```python
from build123d import *

# Parameters (mm, degrees)
F0_W      = 460
F0_H      = 450
F1_DEPTH  = 10
F2_R      = 2.5
F3_DEPTH  = 23
F4_W      = 40
F4_H      = 220
F5_DEPTH  = 160
F6_W      = 380
F6_H      = 25
F7_DEPTH  = 60
F8_W      = 58
F8_H      = 21
F9_DEPTH  = 382.2
F10_DEPTH = 401
F11_W     = 25
F11_H     = 387.5
F12_DEPTH = 60
F13_W     = 21
F13_H     = 58
F14_DEPTH = 386.4
F15_W     = 58
F15_H     = 25
F16_DEPTH = 3.3
F17_W     = 365
F17_H     = 25
F18_DEPTH = 60
F19_W     = 58
F19_H     = 21
F20_DEPTH = 366.6


with BuildPart() as f1:
    # F0 (on Front) → F1 (new body)
    with BuildSketch(Plane.XZ):
        Rectangle(F0_W, F0_H)
    extrude(amount=F1_DEPTH)

    # F2 (on face) → F3 (cut)
    with BuildSketch(Plane.XZ.offset(10)):
        with Locations((210, 205)):
            Circle(F2_R)
        with Locations((-210, 205)):
            Circle(F2_R)
        with Locations((-210, -205)):
            Circle(F2_R)
        with Locations((210, -205)):
            Circle(F2_R)
    extrude(amount=-F3_DEPTH, mode=Mode.SUBTRACT)

    # F4 (on face) → F5 (join)
    with BuildSketch(Plane.XZ.offset(10)):
        with Locations((-195, 60)):
            Rectangle(F4_W, F4_H)
    extrude(amount=F5_DEPTH)

    # F6 (on face) → F7 (join)
    with BuildSketch(Plane.XZ.offset(10)):
        with Locations((0, 202.5)):
            Rectangle(F6_W, F6_H)
        with Locations((0, -202.5)):
            Rectangle(F6_W, F6_H)
    extrude(amount=F7_DEPTH)

    # F8 (on face) → F9 (cut)
    with BuildSketch(Plane.YZ.offset(190)):
        with Locations((-41, 202.5)):
            Rectangle(F8_W, F8_H)
    extrude(amount=-F9_DEPTH, mode=Mode.SUBTRACT)

    # F8 (on face) → F10 (cut)
    with BuildSketch(Plane.YZ.offset(190)):
        with Locations((-41, -202.5)):
            Rectangle(F8_W, F8_H)
    extrude(amount=-F10_DEPTH, mode=Mode.SUBTRACT)

    # F11 (on face) → F12 (join)
    with BuildSketch(Plane.XZ.offset(10)):
        with Locations((210.504704, -3.75)):
            Rectangle(F11_W, F11_H)
    extrude(amount=F12_DEPTH)

    # F13 (on face) → F14 (cut)
    with BuildSketch(Plane(origin=(0, 0, -197.5), x_dir=(1, 0, 0), z_dir=(0, 0, -1))):
        with Locations((210.504704, 41)):
            Rectangle(F13_W, F13_H)
    extrude(amount=-F14_DEPTH, mode=Mode.SUBTRACT)

    # F15 (on face) → F16 (cut)
    with BuildSketch(Plane(origin=(198.004704, 0, 0), x_dir=(0, -1, 0), z_dir=(-1, 0, 0))):
        with Locations((41, -44.218161)):
            Rectangle(F15_W, F15_H)
    extrude(amount=-F16_DEPTH, mode=Mode.SUBTRACT)

    # F17 (on face) → F18 (join)
    with BuildSketch(Plane.XZ.offset(10)):
        with Locations((13.504704, -44.218161)):
            Rectangle(F17_W, F17_H)
    extrude(amount=F18_DEPTH)

    # F19 (on face) → F20 (cut)
    with BuildSketch(Plane.YZ.offset(196.004704)):
        with Locations((-41, -44.218161)):
            Rectangle(F19_W, F19_H)
    extrude(amount=-F20_DEPTH, mode=Mode.SUBTRACT)


solid = f1.part
```
Geometry check sheet. Reference: the model listing, model coordinates, mm. A direction names the side the tool comes from. Give positions to 0.01 mm unless a question says otherwise; leave off trailing zeros. Order: outer loops, then holes, each group sorted by start corner. A loop starts at its lowest first (then second) coordinate and runs counter-clockwise, first axis right, second up. Notation, with made-up numbers: (80, 56.5) - (138, 56.5) arc R28 cw to (138, 83.5) - close; hole circle Ø8 at (27, 66). An arc over 180 degrees is marked (long way). Write item = value, one per line. Start each with the question number.
1) Section check D-D (z = -178). Enter the section's corners in (x, y), then the cut area to 3 significant figures.
2) Scan lines: L1, parallel to Z at x = 19.5, y = -52; L2, parallel to X at y = -26.5, z = 155; L3, parallel to X at y = -3, z = 205. Record each from-to range of solid material in increasing order.
3) Section check B-B (y = -54). Count the separate pieces of the cut face and the enclosed holes in it, then the cut area to 3 significant figures.
4) Access from +Z, -Z, +X, -X, +Y, -Y to the whole of each face (thin tool, end or side, straight path). Record for faces 4 (the flat face through (3, -41, -192)), 5 (the flat face through (198.005, -40, -6)), 6 (the flat face through (3, -41, 213)).
5) Gauge pin test, flat ends, axial feed: pin 1 Ø0.6 at (x, z) = (92.5, 191.5) entering from -Y; pin 2 Ø2 at (x, z) = (-123.5, 51.5) entering from -Y; pin 3 Ø6 at (x, y) = (-120.5, -24) entering from +Z. Record the tip position at first contact, or that the pin passes through.
6) Section check A-A (x = -73). Enter the section's corners in (y, z), then the cut area to 3 significant figures.
7) Draft check along Z on faces 1 (the flat face through (223.005, -40, -6)), 2 (the flat face through (-3, -40, 215)), 3 (the flat face through (-3, -40, -190)). Enter one of: released by +Z, released by -Z, zero draft, split by the parting line, or undercut.
8) Section check C-C (z = 50.5). Enter the section's corners in (x, y).
Geometry check:
q1.outline = (-230, -10) - (198, -10) - (198, -70) - (200, -70) - (200, -12) - (221, -12) - (221, -70) - (223, -70) - (223, -10) - (230, -10) - (230, 0) - (-230, 0) - close
q1.area = 4,880 mm2
q2.L1 = -215 to -213, -192 to -190, -56.72 to -54.72, -33.72 to -31.72, 190 to 192, 213 to 215
q2.L2 = -215 to -175, 198 to 200, 221 to 223
q2.L3 = -230 to -212.5, -207.5 to 207.5, 212.5 to 230
q3.separate_pieces = 9
q3.enclosed_holes = 0
q3.area = 14,800 mm2
q4.face_4 = -X, -Y
q4.face_5 = +Z, -Z, -Y
q4.face_6 = +X, -X, -Y
q5.pin_1 = -70
q5.pin_2 = -10
q5.pin_3 = 215
q6.outline = (-70, -215) - (-10, -215) - (-10, -225) - (0, -225) - (0, 225) - (-10, 225) - (-10, 215) - (-70, 215) - (-70, 213) - (-12, 213) - (-12, 192) - (-70, 192) - (-70, 190) - (-10, 190) - (-10, -31.72) - (-70, -31.72) - (-70, -33.72) - (-12, -33.72) - (-12, -54.72) - (-70, -54.72) - (-70, -56.72) - (-10, -56.72) - (-10, -190) - (-70, -190) - (-70, -192) - (-12, -192) - (-12, -213) - (-70, -213) - close
q6.area = 5,350 mm2
q7.face_1 = zero draft
q7.face_2 = released by +Z
q7.face_3 = undercut
q8.outline = (-230, -10) - (-215, -10) - (-215, -170) - (-175, -170) - (-175, -10) - (198, -10) - (198, -70) - (200, -70) - (200, -12) - (221, -12) - (221, -70) - (223, -70) - (223, -10) - (230, -10) - (230, 0) - (-230, 0) - close
